Check sheet for the modelled part. Datum: model origin and axes. Units: mm. A direction names the side the tool comes from. Give positions to 0.01 mm unless a question says otherwise; leave off trailing zeros. Loops run counter-clockwise (first coordinate to the right, second up) from the corner with the lowest first, then second, coordinate; pieces in that order, holes last. Notation, with made-up numbers: M 44.5,1.25 L 92.5,1.25 A31 cw 92.5,32.25 Z; hole C 85.5,65.5 d6. An arc over 180 degrees is marked long. Write each question's results on one line, items separated by ' | '. Start each with the question number.
1. Sectioned sample at C-C on x = 1.05. Record the cut outline in (y, z), and give its area (3 significant figures).
2. Draft check along Y on faces 1 (the cylindrical face through (1.014, 3.584, -2.285)), 2 (the flat face through (0.99, 6.34, -23.3)), 3 (the cylindrical face through (-0.49, -6.66, 8.69)). Enter one of: pulls with the +Y half, pulls with the -Y half, needs draft (parallel to the pull), parting line crosses it, or undercut.
3. Sectioned sample at A-A on y = 3. Record the cut outline in (x, z), and give its area (3 significant figures).
4. Go/stop test with flat-tipped pins: pin 1 (13.5 mm diameter, centred on y = 0, z = 0, fed in from -X); pin 2 (2.5 mm diameter, centred on y = 0, z = 20, fed in from +X); pin 3 (1 mm diameter, centred on x = 0.5, y = 15, fed in from -Z); pin 4 (1 mm diameter, centred on x = 1, y = -8, fed in from -Z). Record where each tip stops, or that it passes through.
5. Sectioned sample at D-D on z = 6. Record the cut outline in (x, y), and give its area (3 significant figures).
6. Sectioned sample at B-B on z = 19. Record the cut outline in (x, y).
7. Material ranges on line 1 along Y through (x, z) = (1.1, 0); line 2 along Z through (x, y) = (1.85, 1); line 3 along X through (y, z) = (-4.5, -12), recorded low to high.
8. Tool access check on faces 4 (the flat face through (0, -3.2, 3.2)), 5 (the cylindrical face through (1.01, -0.62, 21.97)). Record the directions out of +Z, -Z, +X, -X, +Y, -Y that give a thin tool (end or side, any length) a straight path to the whole face; none if there is none.
Autodesk Inventor part; units mm, degrees
ref_plane "YZ Plane" through (0, 0, 0) normal (1, 0, 0) x (0, 1, 0)
ref_plane "XZ Plane" through (0, 0, 0) normal (0, 1, 0) x (-1, 0, 0)
ref_plane "XY Plane" through (0, 0, 0) normal (0, 0, 1) x (1, 0, 0)
sketch "Esquisse1" plane through (0, 0, 0) normal (1, 0, 0) x (0, 1, 0)
  circle A0 centre (0, 0) radius 10.95
  circle A1 centre (0, 0) radius 25
  line L0 (0, 25) -> (25, 25)
  line L1 (25, 25) -> (25, 0)
  line L2 (21.6506, 12.5) -> (25, 0)
  line L3 (21.6506, 12.5) -> (12.5, 21.6506)
  line L4 (12.5, 21.6506) -> (0, 25)
  line L5 (0, 0) -> (7.9736, 0)
  line L6 (0, 0) -> (0, 6.25)
  line L7 (21.6506, -12.5) -> (25, 0)
  line L8 (21.6506, -12.5) -> (12.5, -21.6506)
  line L9 (12.5, -21.6506) -> (0, -25)
  line L10 (-21.6506, 12.5) -> (-25, 0)
  line L11 (-21.6506, 12.5) -> (-12.5, 21.6506)
  line L12 (-12.5, 21.6506) -> (0, 25)
  line L13 (-21.6506, -12.5) -> (-25, 0)
  line L14 (-21.6506, -12.5) -> (-12.5, -21.6506)
  line L15 (-12.5, -21.6506) -> (0, -25)
  line L16 (-12.5, 21.6506) -> (-12.5, -21.6506)
  arc A2 (-12.5, 21.6506) -> (-12.5, -21.6506) centre (36.4383, 0) ccw
  dimension "d0" = 21.9
  dimension "d1" = 50
extrude "Extrusion1" add sketch "Esquisse1" along normal blind 2 contours L7 L8 L9 L15 L16 L12 L4 L3 L2 | L16 A2
sketch "Esquisse7" plane through (2, 0, 0) normal (1, 0, 0) x (0, 0, -1)
  circle A0 centre (0, 0) radius 10.95
  circle A1 centre (0, 0) radius 4.25
extrude "Extrusion6" add sketch "Esquisse7" against normal blind 3
sketch "Esquisse8" plane through (0, 0, 0) normal (-1, 0, 0) x (0, 0, 1)
  line L0 (0, 0) -> (-20, 0)
  line L1 (0, 0) -> (0, 2.8662)
  point P0 (20, 0)
  dimension "d30" = 20
hole "Perçage2" at (0, 0, -20) at (0, 0, 20) direction (1, 0, 0) diameter 4.134 end through all
sketch "Esquisse9" plane through (-1, 0, 0) normal (-1, 0, 0) x (0, 0, 1)
  circle A0 centre (0, 0) radius 4.25
  circle A1 centre (0, 0) radius 10.95
  circle A2 centre (0, 0) radius 7.5
  dimension "d39" = 15
extrude "Extrusion7" cut sketch "Esquisse9" against normal blind 1 contours A2
properties part number "bielle côté 0"
Output values:
1) outline: M -12.5,-21.65 L 0,-25 L 12.5,-21.65 L 21.65,-12.5 L 25,0 L 21.65,12.5 L 12.5,21.65 L 0,25 L -12.5,21.65 A53.51 ccw Z; hole C 0,0 d8.5; hole C 0,-20 d4.13; hole C 0,20 d4.13 | area: 1,570 mm2
2) face 1: undercut | face 2: pulls with the +Y half | face 3: parting line crosses it
3) outline: M -1,-10.53 L 0,-10.53 L 0,-24.2 L 2,-24.2 L 2,-3.01 L 0,-3.01 L 0,-6.87 L -1,-6.87 Z; M -1,6.87 L 0,6.87 L 0,3.01 L 2,3.01 L 2,24.2 L 0,24.2 L 0,10.53 L -1,10.53 Z | area: 92.1 mm2
4) pin 1: x = 0 | pin 2: through | pin 3: z = -19.65 | pin 4: z = -22.99
5) outline: M -1,-9.16 L 0,-9.16 L 0,-16.74 L 2,-16.74 L 2,23.39 L 0,23.39 L 0,9.16 L -1,9.16 L -1,4.5 L 0,4.5 L 0,-4.5 L -1,-4.5 Z | area: 89.6 mm2
6) outline: M 0,-13.59 L 2,-13.59 L 2,-1.81 L 0,-1.81 Z; M 0,1.81 L 2,1.81 L 2,15.15 L 0,15.15 Z
7) line 1: -17.08 to -4.25, 4.25 to 25 | line 2: -24.73 to -21.81, -18.19 to -4.13, 4.13 to 18.19, 21.81 to 24.73 | line 3: 0 to 2
8) face 4: -X | face 5: +X, -X
